For this review, use the dimensioned drawing (mm, ordinates from the lowest corner) and the shaded views. Give positions to 0.01 mm unless a question says otherwise; leave off trailing zeros. Loops run counter-clockwise (first coordinate to the right, second up) from the corner with the lowest first, then second, coordinate; pieces in that order, holes last. Notation, with made-up numbers: M 8.25,56.5 L 15.25,56.5 A21 ccw 15.25,62.5 Z; hole C -23.75,28.5 d4. An arc over 180 degrees is marked long. Use CSV: the item, a comma, the result in double quotes.
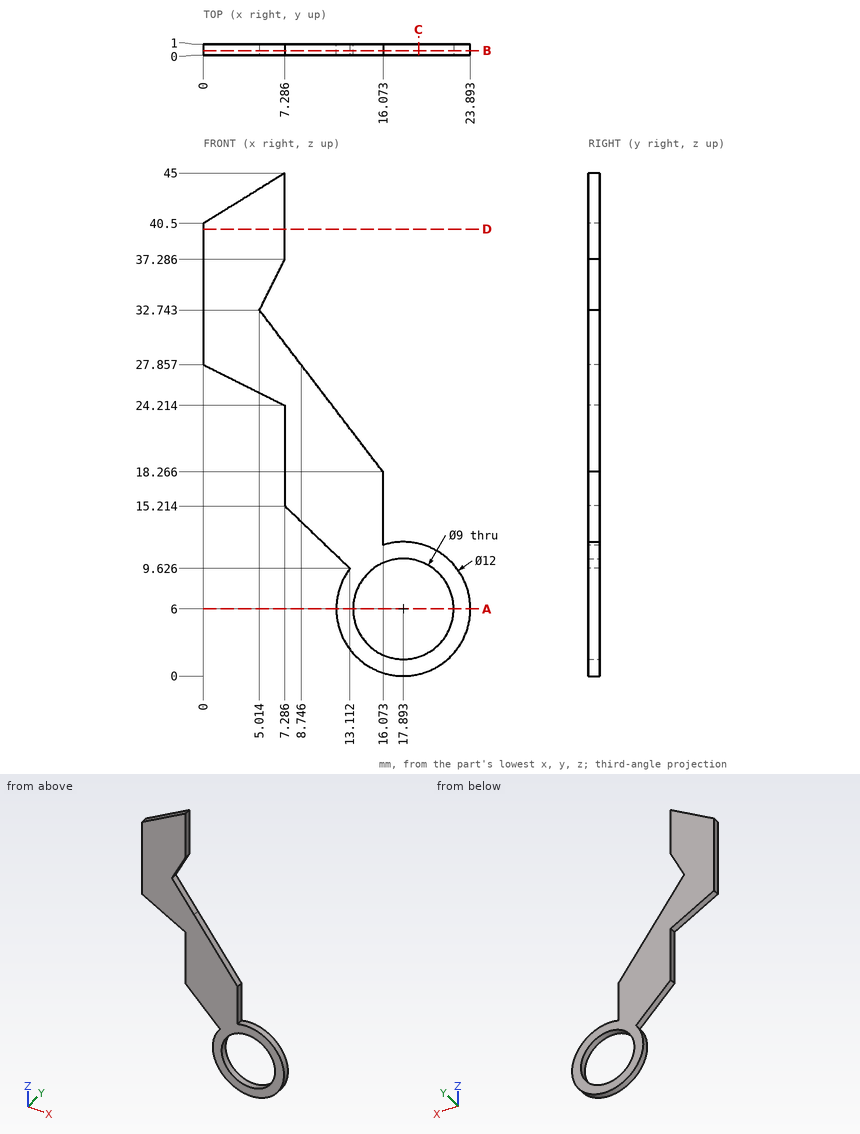
(1) We need section B-B on y = 0.4. State the section outline as (x, z) points (1 decimal).
A:
outline,"M 0,27.9 L 7.3,24.2 L 7.3,15.2 L 13.1,9.6 A6 ccw long 16.1,11.7 L 16.1,18.3 L 8.7,27.9 L 5,32.7 L 7.3,37.3 L 7.3,45 L 0,40.5 Z; hole C 17.9,6 d9"
(2) Wall thickness on line 1 along X through (y, z) = (0.2, 6); line 2 along Z through (x, y) = (13, 0.1) (1 decimal); line 3 along Z through (x, y) = (6.25, 0.7) (1 decimal): over which ranges is each line inside the solid? List them lowest first. Write a range as [from, to].
A:
line 1,"[11.89, 13.39], [22.39, 23.89]"
line 2,"[2.5, 9.5], [9.7, 22.3]"
line 3,"[24.7, 31.1], [35.2, 44.4]"
(3) We need section A-A on z = 6. State the section outline as (x, y) points.
A:
outline,"M 11.89,0 L 13.39,0 L 13.39,1 L 11.89,1 Z; M 22.39,0 L 23.89,0 L 23.89,1 L 22.39,1 Z"
(4) We need section D-D on z = 40. State the section outline as (x, y) points (1 decimal).
A:
outline,"M 0,0 L 7.3,0 L 7.3,1 L 0,1 Z"
(5) We need section C-C on x = 19.25. State the section outline as (y, z) points (1 decimal).
A:
outline,"M 0,0.2 L 1,0.2 L 1,1.7 L 0,1.7 Z; M 0,10.3 L 1,10.3 L 1,11.8 L 0,11.8 Z"
(6) Clearance check with flat-ended pins moving along their axes: P1, Ø5.5, axis at x = 17.89, z = 6, coming from the -Y side; P2, Ø0.5, axis at y = 0.5, z = 22, coming from the -X side. State where each tip first meets the part, or that it passes through.
A:
P1,"through"
P2,"x = 7.29"
